Input: part model. Units: mm. Frame: model coordinates. A direction names the side the tool comes from. Coordinates: 2 decimals unless noted, no trailing zeros. Write each loop counter-clockwise with the first axis right and the second up, starting at its lowest first coordinate (ties: lowest second). Pieces come first, ordered by that corner, then holes.
1) Set-up query: faces 1 (the flat face through (-239.118, 1.268, -13.897)), 2 (the flat face through (-209, 1, 0)). Return all of +Z, -Z, +X, -X, +Y, -Y with unobstructed straight access to the full face (end or side cutting, diameter ignored); none if empty.
2) Section query B-B (y = 0.9). Output: boundary loops of the cut face in (x, z), then the cut area to 3 significant figures.
3) Section query A-A (z = -13.5). Output: boundary loops of the cut face in (x, y).
4) Pin query (flat end, axial travel): pin 1 Ø1.5 at (y, z) = (2, -21) entering from -X; pin 2 Ø3 at (x, z) = (-262.5, -18.5) entering from -Y; pin 3 Ø1 at (y, z) = (2, -13) entering from +X. Return the tip coordinate at first contact, or that it passes through.
5) Section query C-C (x = -225.5). Output: boundary loops of the cut face in (y, z).
6) Section query D-D (x = -262.5). Output: boundary loops of the cut face in (y, z), then the cut area to 3 significant figures.
7) Line query: L1, parallel to Z at x = -169, y = 0.7; L2, parallel to Z at x = -228.5, y = 1.95; L3, parallel to X at y = 1.9, z = -17. Output: solid intervals per line, ascending.
Autodesk Inventor part; units mm, degrees
ref_plane "YZ Plane" through (0, 0, 0) normal (1, 0, 0) x (0, 1, 0)
ref_plane "XZ Plane" through (0, 0, 0) normal (0, 1, 0) x (-1, 0, 0)
ref_plane "XY Plane" through (0, 0, 0) normal (0, 0, 1) x (1, 0, 0)
sketch "スケッチ1" plane through (0, 0, 0) normal (0, 1, 0) x (-1, 0, 0)
  circle A0 centre (0, 0) radius 178.1675
  circle A1 centre (0, 0) radius 157.8276
  line L0 (168.1877, 0) -> (166.7488, -21.9529)
  line L1 (168.1877, 0) -> (130.1721, 2.4917) construction
  line L2 (249.4344, 0) -> (-249.4344, 0)
  line L3 (166.7488, -21.9529) -> (156.7702, -21.2989)
  line L4 (156.7702, -21.2989) -> (158.2091, 0.654) construction
  line L5 (158.2091, 0.654) -> (168.1877, 0)
  line L6 (157.4896, -10.3224) -> (0, 0)
  line L7 (166.7488, -21.9529) -> (162.4568, -43.5302)
  line L8 (162.4568, -43.5302) -> (152.649, -41.5793) construction
  line L9 (152.649, -41.5793) -> (156.9409, -20.002) construction
  line L10 (156.9409, -20.002) -> (166.7488, -21.9529) construction
  line L11 (162.4568, -43.5302) -> (155.3851, -64.3626)
  line L12 (155.3851, -64.3626) -> (145.9158, -61.1482) construction
  line L13 (145.9158, -61.1482) -> (152.9875, -40.3158) construction
  line L14 (152.9875, -40.3158) -> (162.4568, -43.5302) construction
  line L15 (155.3851, -64.3626) -> (145.6548, -84.0938)
  line L16 (145.6548, -84.0938) -> (136.6861, -79.6709) construction
  line L17 (136.6861, -79.6709) -> (146.4164, -59.9397) construction
  line L18 (146.4164, -59.9397) -> (155.3851, -64.3626) construction
  line L19 (0, 0) -> (111.6009, -111.6009)
  line L20 (145.6548, -84.0938) -> (137.3401, -78.5381) construction
  line L21 (137.3401, -78.5381) -> (125.1176, -96.8305) construction
  line L22 (125.1176, -96.8305) -> (133.4323, -102.3862) construction
  line L23 (133.4323, -102.3862) -> (145.6548, -84.0938)
  line L24 (133.4323, -102.3862) -> (125.9139, -95.7927) construction
  line L25 (125.9139, -95.7927) -> (111.4082, -112.3332) construction
  line L26 (111.4082, -112.3332) -> (118.9266, -118.9266)
  line L27 (118.9266, -118.9266) -> (133.4323, -102.3862)
  line L28 (111.6009, -111.6009) -> (118.9266, -118.9266)
  line L29 (166.7488, -21.9529) -> (176.7274, -22.6069) construction
  line L30 (118.9266, -118.9266) -> (125.9834, -125.9834)
  point P0 (154.795, -30.7906)
  point P1 (149.4517, -50.732)
  point P2 (141.5512, -69.8053)
  point P3 (131.2288, -87.6843)
  point P4 (118.661, -104.0629)
  point P5 (157.8276, 0)
  point P6 (178.1675, 0)
  dimension "d0" = 22
  dimension "d1" = 10
  dimension "d2" = 45
  dimension "d4" = 315.6551
extrude "押し出し1" add sketch "スケッチ1" along normal blind 2.5 contours L30 L27 L23 L15 L11 L7 L0 L2 A0 | L28 A1 L2 L0 L7 L11 L15 L23 L27
sketch "スケッチ2" plane through (0, 2.5, 0) normal (0, 1, 0) x (1, 0, 0)
  circle A0 centre (0, 0) radius 277.8276
  line L0 (-168.1877, 0) -> (-166.7488, 21.9529)
  line L1 (-166.7488, 21.9529) -> (-162.4568, 43.5302)
  line L2 (-162.4568, 43.5302) -> (-155.3851, 64.3626)
  line L3 (-155.3851, 64.3626) -> (-145.6548, 84.0938)
  line L4 (-133.4323, 102.3862) -> (-145.6548, 84.0938)
  line L5 (-118.9266, 118.9266) -> (-133.4323, 102.3862)
  line L6 (-167.4682, 10.9764) -> (-166.0294, 32.9293)
  line L7 (-166.0294, 32.9293) -> (-275.7938, 40.1237)
  line L8 (-275.7938, 40.1237) -> (-277.2327, 18.1708)
  line L9 (-277.2327, 18.1708) -> (-167.4682, 10.9764)
  line L10 (-164.6028, 32.7415) -> (-160.3108, 54.3188)
  line L11 (-160.3108, 54.3188) -> (-268.1972, 75.7787)
  line L12 (-268.1972, 75.7787) -> (-272.4892, 54.2015)
  line L13 (-272.4892, 54.2015) -> (-164.6028, 32.7415)
  circle A1 centre (-166.7488, 21.9529) radius 11
  circle A2 centre (-162.4568, 43.5302) radius 11
  line L14 (-158.921, 53.9464) -> (-151.8493, 74.7789)
  line L15 (-151.8493, 74.7789) -> (-256.0116, 110.1372)
  line L16 (-256.0116, 110.1372) -> (-263.0833, 89.3047)
  line L17 (-263.0833, 89.3047) -> (-158.921, 53.9464)
  circle A3 centre (-155.3851, 64.3626) radius 11
  arc A4 (-275.7591, 62.4834) -> (-281.3553, 41.7349) centre (-166.7488, 21.9529) ccw
  line L18 (-178.1663, 0.654) -> (-158.2091, -0.654)
  line L19 (-158.2091, -0.654) -> (-156.7702, 21.2989)
  line L20 (-156.7702, 21.2989) -> (-176.7274, 22.6069)
  line L21 (-176.7274, 22.6069) -> (-178.1663, 0.654)
  line L22 (-177.4468, 11.6305) -> (-275.7938, 40.1237)
  line L23 (-176.7274, 22.6069) -> (-176.008, 33.5834)
  line L24 (-176.008, 33.5834) -> (-275.7591, 62.4834)
  line L25 (-275.7938, 40.1237) -> (-281.3553, 41.7349)
  circle A5 centre (0, 0) radius 137.8276
  line L26 (0, 0) -> (-196.4538, 196.4538)
  line L27 (-111.6009, 111.6009) -> (-125.9834, 125.9834)
  line L28 (-411.1762, 0) -> (411.1762, 0)
  circle A6 centre (0, 0) radius 257.8276 construction
  arc A7 (-111.6009, 111.6009) -> (-157.8276, 0) centre (0, 0) ccw
  point P0 (-158.1662, 0)
  point P1 (-137.8276, 0)
  point P2 (-97.4588, 97.4588)
  point P3 (-277.8276, 0)
  dimension "d7" = 22
  dimension "d10" = 20
  dimension "d11" = 100
  dimension "d12" = 20
  dimension "d14" = 20
  dimension "d17" = 100
extrude "押し出し2" add sketch "スケッチ2" against normal blind 2.5 contours L26 L5 L4 L3 A3 L15 A0 | A0 L9 L21 L18 L28 | L15 A3 L17 A0 | A0 L22 L9 | L18 L21 L9 L0 | L0 A1 L19 L28 | A5 L28 A7 A1 A2 A3 L26 | L17 A2 L11 A0 | A3 L3 L14 | L14 L2 A3 | L26 A7 A3 L3 L4 L5 | A0 L7 L23 A1 L21 L22 | L21 A1 L9 | A1 L21 L20 L0 | L0 L20 L19 A1 | L19 A7 L28 | L11 A2 L13 L24 A0 | A2 A7 L1 L2 | L2 L10 A2 | A3 A7 A2 | L2 L3 A3 A7 | A0 L13 L24 L7 | A1 L23 L21 | L6 A1 L1 | L20 L23 A1 L6 | L1 A1 A7 L19 L20 | A1 A7 L19 | A3 A7 | L24 L13 A0 | L10 L1 A2 | A2 A7 | L24 L13 A1 L7 | L7 A1 L23 | A2 A7 A1 | A7 A1
sketch "スケッチ4" plane through (0, 2.5, 0) normal (0, 1, 0) x (1, 0, 0)
  circle A0 centre (0, 0) radius 187.8276
  arc A1 (-97.4588, 97.4588) -> (-137.8276, 0) centre (0, 0) ccw
  line L0 (-137.5954, 7.9966) -> (-277.3596, 16.1193)
  line L1 (-137.5954, 7.9966) -> (-137.8276, 0)
  arc A2 (-196.4538, 196.4538) -> (-277.8276, 0) centre (0, 0) ccw
  line L2 (-137.8276, 0) -> (-128.5432, -0.2696)
  line L3 (-185.8501, 27.1836) -> (-136.3765, 19.9473)
  line L4 (-136.3765, 19.9473) -> (-137.8276, 0)
  line L5 (-120.1573, -1.2854) -> (-137.8276, 0)
  line L6 (-97.4588, 97.4588) -> (-196.4538, 196.4538)
  point P0 (-187.5112, 10.8976)
  dimension "d23" = 50
  dimension "d24" = 8
  dimension "d25" = 20
extrude "押し出し4" cut sketch "スケッチ4" against normal through all contours L6 A1 L3 A0 | A0 L0 A2 L6
fillet "フィレット2" radius 15 1 edges at (-187.5112, 1.25, -10.8976)
properties material "木材 (カエデ材)"
Answer:
1. face 1: -Z, +Y, -Y
1. face 2: +Z, +X, -X, +Y, -Y
2. outline: (-277.83, 0) arc R277.83 ccw to (-277.36, -16.12) - (-201.93, -11.74) arc R15 cw to (-186.19, -24.74) arc R187.83 ccw to (-185.85, -27.18) - (-136.38, -19.95) arc R137.83 cw to (-137.83, 0) - close
2. area: 2,440 mm2
3. outline: (-277.5, 0) - (-232.29, 0) - (-232.29, 2.5) - (-277.5, 2.5) - close; (-193.96, 0) - (-137.16, 0) - (-137.16, 2.5) - (-193.96, 2.5) - close
4. pin 1: stops at x = -187.52
4. pin 2: passes through
4. pin 3: stops at x = -137.16
5. outline: (0, -13.11) - (2.5, -13.11) - (2.5, 0) - (0, 0) - close
6. outline: (0, -15.26) - (2.5, -15.26) - (2.5, 0) - (0, 0) - close
6. area: 38.1 mm2
7. L1: z = -24.72 to 0
7. L2: z = -13.28 to 0
7. L3: x = -189.63 to -136.78
